Design review of the part built by this model. Coordinates are the model's own, in mm. Coordinates: 2 decimals unless noted, no trailing zeros. Write each loop counter-clockwise with the first axis right and the second up, starting at its lowest first coordinate (ties: lowest second). Pieces come first, ordered by that corner, then holes.
Q1. Add section B-B, the plane y = 2.5. Give the number of separate pieces and of enclosed holes in the cut face, plus the area to 3 significant figures.
Q2. Add section A-A, the plane z = 0. Give the boundary of the cut face in (x, y), plus the area to 3 significant figures.
Q3. Add section D-D, the plane z = 26. Give the boundary of the cut face in (x, y).
Q4. Clearance check with flat-ended pins moving along their axes: pin 1 Ø3 at (x, z) = (14.8, -73.1) entering from -Y; pin 2 Ø1.2 at (x, y) = (62, 3.5) entering from +Z; pin 3 Ø1.5 at (y, z) = (3.5, -2.5) entering from -X; pin 4 Ø2 at (x, y) = (63, 3) entering from -Z. State where each tip first meets the part, or that it passes through.
Q5. To check wall thickness, follow probe 1 along X at (y, z) = (4.75, -0.5); probe 2 along Z at (x, y) = (-14.8, 2.9); probe 3 along X at (y, z) = (4.85, -50.5). State the ranges of each line that lie inside material, in increasing order.
Q6. Add section C-C, the plane x = -52.5. Give the boundary of the cut face in (y, z).
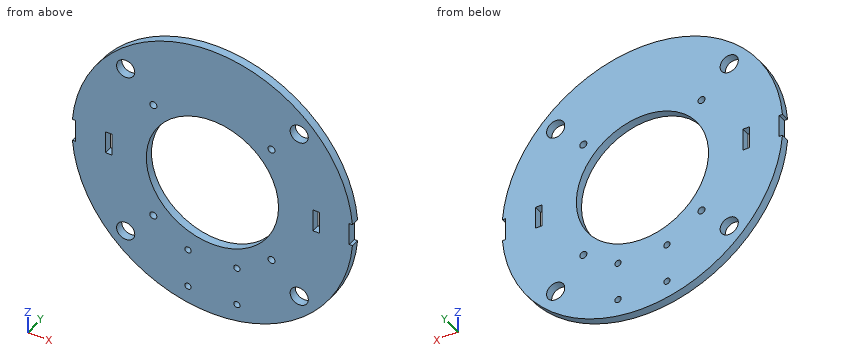
from build123d import *

# Parameters (mm, degrees)
SKETCH1_R               = 85
BASE_DEPTH              = 5
MAIN_WHEEL_SLOTS_REACH  = 7
SKETCH2_W               = 4
SKETCH2_H               = 13.5
F_3RD_WHEEL_HOLES_REACH = 7
SKETCH3_R               = 1.9
SKETCH6_R               = 2.15
FAN_SCREW_HOLES_DEPTH   = 6
SKETCH7_R               = 40
FAN_BLADE_HOLE_DEPTH    = 6
BOLT_HOLES_REACH        = 7
SKETCH8_R               = 5.5


with BuildPart() as part:
    # Sketch1 → Base (new body)
    with BuildSketch(Plane(origin=(0, 0, 0), x_dir=(1, 0, 0), z_dir=(0, 1, 0))):
        Circle(SKETCH1_R)
    extrude(amount=BASE_DEPTH)

    # Sketch2 → Main Wheel Slots (cut, up to next)
    with BuildSketch(Plane(origin=(0, 5, 0), x_dir=(1, 0, 0), z_dir=(0, 1, 0)), mode=Mode.PRIVATE) as main_wheel_slots_sk1:
        with Locations((62.731561416, 0)):
            Rectangle(SKETCH2_W, SKETCH2_H)
    main_wheel_slots_tool1 = extrude(main_wheel_slots_sk1.sketch, amount=-MAIN_WHEEL_SLOTS_REACH, mode=Mode.PRIVATE) & part.part
    add(main_wheel_slots_tool1.solids().sort_by_distance((62.731561, 5, 0))[0], mode=Mode.SUBTRACT)
    # Sketch2 → Main Wheel Slots (cut, up to next)
    with BuildSketch(Plane(origin=(0, 5, 0), x_dir=(1, 0, 0), z_dir=(0, 1, 0)), mode=Mode.PRIVATE) as main_wheel_slots_sk2:
        with BuildLine():
            ThreePointArc((85, 0), (84.932863841, 3.377667808), (84.731561416, 6.75))
            Line((84.731561416, 6.75), (82.731561416, 6.75))
            Line((82.731561416, 6.75), (82.731561416, -6.75))
            Line((82.731561416, -6.75), (84.731561416, -6.75))
            ThreePointArc((84.731561416, -6.75), (84.932863841, -3.377667808), (85, 0))
        make_face()
    main_wheel_slots_tool2 = extrude(main_wheel_slots_sk2.sketch, amount=-MAIN_WHEEL_SLOTS_REACH, mode=Mode.PRIVATE) & part.part
    add(main_wheel_slots_tool2.solids().sort_by_distance((83.822538, 5, 0))[0], mode=Mode.SUBTRACT)
    # Sketch2 → Main Wheel Slots (cut, up to next)
    with BuildSketch(Plane(origin=(0, 5, 0), x_dir=(1, 0, 0), z_dir=(0, 1, 0)), mode=Mode.PRIVATE) as main_wheel_slots_sk3:
        with BuildLine():
            Line((-82.731561416, 6.75), (-84.731561416, 6.75))
            ThreePointArc((-84.731561416, 6.75), (-85, 0), (-84.731561416, -6.75))
            Line((-84.731561416, -6.75), (-82.731561416, -6.75))
            Line((-82.731561416, -6.75), (-82.731561416, 6.75))
        make_face()
    main_wheel_slots_tool3 = extrude(main_wheel_slots_sk3.sketch, amount=-MAIN_WHEEL_SLOTS_REACH, mode=Mode.PRIVATE) & part.part
    add(main_wheel_slots_tool3.solids().sort_by_distance((-83.822538, 5, 0))[0], mode=Mode.SUBTRACT)
    # Sketch2 → Main Wheel Slots (cut, up to next)
    with BuildSketch(Plane(origin=(0, 5, 0), x_dir=(1, 0, 0), z_dir=(0, 1, 0)), mode=Mode.PRIVATE) as main_wheel_slots_sk4:
        with Locations((-62.731561416, 0)):
            Rectangle(SKETCH2_W, SKETCH2_H)
    main_wheel_slots_tool4 = extrude(main_wheel_slots_sk4.sketch, amount=-MAIN_WHEEL_SLOTS_REACH, mode=Mode.PRIVATE) & part.part
    add(main_wheel_slots_tool4.solids().sort_by_distance((-62.731561, 5, 0))[0], mode=Mode.SUBTRACT)

    # Sketch3 → 3rd Wheel Holes (cut, up to next)
    with BuildSketch(Plane(origin=(0, 5, 0), x_dir=(1, 0, 0), z_dir=(0, 1, 0)), mode=Mode.PRIVATE) as f_3rd_wheel_holes_sk1:
        with Locations((14.8, 73.1)):
            Circle(SKETCH3_R)
    f_3rd_wheel_holes_tool1 = extrude(f_3rd_wheel_holes_sk1.sketch, amount=-F_3RD_WHEEL_HOLES_REACH, mode=Mode.PRIVATE) & part.part
    add(f_3rd_wheel_holes_tool1.solids().sort_by_distance((14.8, 5, -73.1))[0], mode=Mode.SUBTRACT)
    # Sketch3 → 3rd Wheel Holes (cut, up to next)
    with BuildSketch(Plane(origin=(0, 5, 0), x_dir=(1, 0, 0), z_dir=(0, 1, 0)), mode=Mode.PRIVATE) as f_3rd_wheel_holes_sk2:
        with Locations((14.8, 49.6)):
            Circle(SKETCH3_R)
    f_3rd_wheel_holes_tool2 = extrude(f_3rd_wheel_holes_sk2.sketch, amount=-F_3RD_WHEEL_HOLES_REACH, mode=Mode.PRIVATE) & part.part
    add(f_3rd_wheel_holes_tool2.solids().sort_by_distance((14.8, 5, -49.6))[0], mode=Mode.SUBTRACT)
    # Sketch3 → 3rd Wheel Holes (cut, up to next)
    with BuildSketch(Plane(origin=(0, 5, 0), x_dir=(1, 0, 0), z_dir=(0, 1, 0)), mode=Mode.PRIVATE) as f_3rd_wheel_holes_sk3:
        with Locations((-14.8, 49.6)):
            Circle(SKETCH3_R)
    f_3rd_wheel_holes_tool3 = extrude(f_3rd_wheel_holes_sk3.sketch, amount=-F_3RD_WHEEL_HOLES_REACH, mode=Mode.PRIVATE) & part.part
    add(f_3rd_wheel_holes_tool3.solids().sort_by_distance((-14.8, 5, -49.6))[0], mode=Mode.SUBTRACT)
    # Sketch3 → 3rd Wheel Holes (cut, up to next)
    with BuildSketch(Plane(origin=(0, 5, 0), x_dir=(1, 0, 0), z_dir=(0, 1, 0)), mode=Mode.PRIVATE) as f_3rd_wheel_holes_sk4:
        with Locations((-14.8, 73.1)):
            Circle(SKETCH3_R)
    f_3rd_wheel_holes_tool4 = extrude(f_3rd_wheel_holes_sk4.sketch, amount=-F_3RD_WHEEL_HOLES_REACH, mode=Mode.PRIVATE) & part.part
    add(f_3rd_wheel_holes_tool4.solids().sort_by_distance((-14.8, 5, -73.1))[0], mode=Mode.SUBTRACT)

    # Sketch6 → Fan Screw Holes (cut)
    with BuildSketch(Plane(origin=(0, 5, 0), x_dir=(1, 0, 0), z_dir=(0, 1, 0))):
        with Locations((35.75, 35.75)):
            Circle(SKETCH6_R)
        with Locations((-35.75, 35.75)):
            Circle(SKETCH6_R)
        with Locations((35.75, -35.75)):
            Circle(SKETCH6_R)
        with Locations((-35.75, -35.75)):
            Circle(SKETCH6_R)
    extrude(amount=-FAN_SCREW_HOLES_DEPTH, mode=Mode.SUBTRACT)

    # Sketch7 → Fan Blade Hole (cut)
    with BuildSketch(Plane(origin=(0, 5, 0), x_dir=(1, 0, 0), z_dir=(0, 1, 0))):
        Circle(SKETCH7_R)
    extrude(amount=-FAN_BLADE_HOLE_DEPTH, mode=Mode.SUBTRACT)

    # Sketch8 → Bolt Holes (cut, up to next)
    with BuildSketch(Plane(origin=(0, 5, 0), x_dir=(1, 0, 0), z_dir=(0, 1, 0)), mode=Mode.PRIVATE) as bolt_holes_sk1:
        with Locations((52.5, 52.5)):
            Circle(SKETCH8_R)
    bolt_holes_tool1 = extrude(bolt_holes_sk1.sketch, amount=-BOLT_HOLES_REACH, mode=Mode.PRIVATE) & part.part
    add(bolt_holes_tool1.solids().sort_by_distance((52.5, 5, -52.5))[0], mode=Mode.SUBTRACT)
    # Sketch8 → Bolt Holes (cut, up to next)
    with BuildSketch(Plane(origin=(0, 5, 0), x_dir=(1, 0, 0), z_dir=(0, 1, 0)), mode=Mode.PRIVATE) as bolt_holes_sk2:
        with Locations((-52.5, 52.5)):
            Circle(SKETCH8_R)
    bolt_holes_tool2 = extrude(bolt_holes_sk2.sketch, amount=-BOLT_HOLES_REACH, mode=Mode.PRIVATE) & part.part
    add(bolt_holes_tool2.solids().sort_by_distance((-52.5, 5, -52.5))[0], mode=Mode.SUBTRACT)
    # Sketch8 → Bolt Holes (cut, up to next)
    with BuildSketch(Plane(origin=(0, 5, 0), x_dir=(1, 0, 0), z_dir=(0, 1, 0)), mode=Mode.PRIVATE) as bolt_holes_sk3:
        with Locations((52.5, -52.5)):
            Circle(SKETCH8_R)
    bolt_holes_tool3 = extrude(bolt_holes_sk3.sketch, amount=-BOLT_HOLES_REACH, mode=Mode.PRIVATE) & part.part
    add(bolt_holes_tool3.solids().sort_by_distance((52.5, 5, 52.5))[0], mode=Mode.SUBTRACT)
    # Sketch8 → Bolt Holes (cut, up to next)
    with BuildSketch(Plane(origin=(0, 5, 0), x_dir=(1, 0, 0), z_dir=(0, 1, 0)), mode=Mode.PRIVATE) as bolt_holes_sk4:
        with Locations((-52.5, -52.5)):
            Circle(SKETCH8_R)
    bolt_holes_tool4 = extrude(bolt_holes_sk4.sketch, amount=-BOLT_HOLES_REACH, mode=Mode.PRIVATE) & part.part
    add(bolt_holes_tool4.solids().sort_by_distance((-52.5, 5, 52.5))[0], mode=Mode.SUBTRACT)


solid = part.part
Here are the results:
1. separate pieces: 1
1. enclosed holes: 15
1. area: 17,000 mm2
2. outline: (-82.73, 0) - (-64.73, 0) - (-64.73, 5) - (-82.73, 5) - close; (-60.73, 0) - (-40, 0) - (-40, 5) - (-60.73, 5) - close; (40, 0) - (60.73, 0) - (60.73, 5) - (40, 5) - close; (64.73, 0) - (82.73, 0) - (82.73, 5) - (64.73, 5) - close
2. area: 387 mm2
3. outline: (-80.93, 0) - (-30.4, 0) - (-30.4, 5) - (-80.93, 5) - close; (30.4, 0) - (80.93, 0) - (80.93, 5) - (30.4, 5) - close
4. pin 1: passes through
4. pin 2: stops at z = 58.78
4. pin 3: stops at x = -82.73
4. pin 4: stops at z = -58.15
5. probe 1: x = -82.73 to -64.73, -60.73 to -40, 40 to 60.73, 64.73 to 82.73
5. probe 2: z = -83.7 to -75, -71.2 to -51.5, -47.7 to -37.16, 37.16 to 83.7
5. probe 3: x = -68.37 to -57.62, -47.38 to -16.47, -13.13 to 13.13, 16.47 to 47.38, 57.62 to 68.37
6. outline: (0, -66.85) - (5, -66.85) - (5, -58) - (0, -58) - close; (0, -47) - (5, -47) - (5, 47) - (0, 47) - close; (0, 58) - (5, 58) - (5, 66.85) - (0, 66.85) - close
